Work out the finished part from the listing and answer in its coordinate system (mm). A direction names the side the tool comes from. Coordinates: 2 decimals unless noted, no trailing zeros. Order: outer loops, then holes, each group sorted by start corner. A loop starts at its lowest first (then second) coordinate and runs counter-clockwise, first axis right, second up. Notation, with made-up numbers: M 36.5,43 L 47.5,43 A12 ccw 47.5,53 Z; hole C 51,71 d3. An arc over 180 degrees is marked long. Use a Markdown table: item, result.
from build123d import *

# Parameters (mm, degrees)
BODY_DEPTH     = 8.5
SKETCH2_W      = 13
SKETCH2_H      = 14
EXTUSION_DEPTH = 15
SKETCH3_W      = 4
SKETCH3_H      = 6
HOLE_A_DEPTH   = 25.212600026
SKETCH4_W      = 4
SKETCH4_H      = 6
HOLE_B_DEPTH   = 17


with BuildPart() as part:
    # Sketch1 → Body (new, symmetric)
    with BuildSketch(Plane(origin=(0, 0, 0), x_dir=(0, 0, -1), z_dir=(1, 0, 0))):
        Polygon((3, 17), (0, 17), (0, 0), (17, 0), (17, 3), align=None)
    extrude(amount=BODY_DEPTH, both=True)

    # Sketch2 → Extusion (cut)
    with BuildSketch(Plane(origin=(0, 0, -17), x_dir=(-1, 0, 0), z_dir=(0, 0, -1))):
        with Locations((0, 10)):
            Rectangle(SKETCH2_W, SKETCH2_H)
    extrude(amount=-EXTUSION_DEPTH, mode=Mode.SUBTRACT)

    # Sketch3 → Hole_A (cut, through all)
    with BuildSketch(Plane(origin=(0, 0, -2), x_dir=(-1, 0, 0), z_dir=(0, 0, -1))):
        with Locations((0, 11)):
            Rectangle(SKETCH3_W, SKETCH3_H)
    extrude(amount=-HOLE_A_DEPTH, mode=Mode.SUBTRACT)

    # Sketch4 → Hole_B (cut)
    with BuildSketch(Plane(origin=(0, 3, 0), x_dir=(1, 0, 0), z_dir=(0, 1, 0))):
        with Locations((0, 11)):
            Rectangle(SKETCH4_W, SKETCH4_H)
    extrude(amount=-HOLE_B_DEPTH, mode=Mode.SUBTRACT)


solid = part.part
1. Section C-C on z = -13.75 is taken. Determine the outline of the cut face in (x, y), then the cut area to 3 significant figures.
Answers below:
| item | result |
|---|---|
| outline | M -8.5,0 L -2,0 L -2,3 L -6.5,3 L -6.5,6.25 L -8.5,6.25 Z; M 2,0 L 8.5,0 L 8.5,6.25 L 6.5,6.25 L 6.5,3 L 2,3 Z |
| area | 52.0 mm² |
2. Section D-D on z = -2.5 is taken. Determine the outline of the cut face in (x, y).
Answers below:
| item | result |
|---|---|
| outline | M -8.5,0 L 8.5,0 L 8.5,17 L 6.5,17 L 6.5,3 L -6.5,3 L -6.5,17 L -8.5,17 Z |
3. For a pull along Z with two mould halves and no side action, classify faces 5 (the face through (-6.5, 8, -8)), 6 (the face through (-2, 2, -11)), 7 (the face through (0, 2, -14)), 8 (the face through (0, 1, -17)) as +Z half, -Z half, draft (parallel to the pull), parting line (faces both ways), or undercut.
Answers below:
| item | result |
|---|---|
| face 5 | draft |
| face 6 | undercut |
| face 7 | undercut |
| face 8 | -Z half |
4. Find the intervals of material crossed by probe 1 along X at (y, z) = (3.25, -5.25); probe 2 along Y at (x, z) = (4.25, -6); probe 3 along Z at (x, y) = (3.75, 9), in increasing order.
Answers below:
| item | result |
|---|---|
| probe 1 | -8.5 to -6.5, 6.5 to 8.5 |
| probe 2 | 0 to 3 |
| probe 3 | -2 to 0 |
5. Section A-A on y = 13.25 is taken. Determine the outline of the cut face in (x, z).
Answers below:
| item | result |
|---|---|
| outline | M -8.5,-6.75 L -6.5,-6.75 L -6.5,-2 L -2,-2 L -2,0 L -8.5,0 Z; M 2,-2 L 6.5,-2 L 6.5,-6.75 L 8.5,-6.75 L 8.5,0 L 2,0 Z |
6. For faces 1 (the face through (0, 2, -8)), 2 (the face through (3, 3, -10)), 3 (the face through (-2, 11, -1)), 4 (the face through (0, 0, -6)), determine the directions among +Z, -Z, +X, -X, +Y, -Y from which every point of the face is accessible in a straight line to the end or side of a thin tool.
Answers below:
| item | result |
|---|---|
| face 1 | +Y, -Y |
| face 2 | -Z, +Y |
| face 3 | +Z, -Z |
| face 4 | +Z, -Z, +X, -X, -Y |
7. Flat-ended cylindrical pins translate along their axes: P1, Ø1.5, axis at x = -6, z = -7, coming from the +Y side; P2, Ø1, axis at x = 4, z = -12, coming from the +Y side. Find the tip coordinate at first contact, or state that the pin passes through.
Answers below:
| item | result |
|---|---|
| P1 | y = 13.56 |
| P2 | y = 3 |
8. Section B-B on x = 1.75 is taken. Determine the outline of the cut face in (y, z).
Answers below:
| item | result |
|---|---|
| outline | M 0,-17 L 3,-17 L 3,-14 L 0,-14 Z; M 0,-8 L 3,-8 L 3,-2 L 8,-2 L 8,0 L 0,0 Z; M 14,-2 L 17,-2 L 17,0 L 14,0 Z |
